The drawing under review shows one solid part. Ordinate dimensions are in mm from its lowest x, y, z. A direction names the side the tool comes from. Coordinates: 2 decimals unless noted, no trailing zeros. Order: outer loops, then holes, each group sorted by start corner. A loop starts at its lowest first (then second) coordinate and runs counter-clockwise, first axis right, second up. Notation, with made-up numbers: (31, -23.75) -> (60, -23.75) arc R8 cw to (60, -8.75) -> close; hole circle Ø11 at (16, 11). An arc over 180 degrees is marked (long way). Use a Markdown table: item, result. Add a question column.
Q1. Add section C-C (x = 24.5). State the section outline as (y, z) points.
Q2. Machinability: for the marked faces 1, 2, 3, 4 and 5, which of the approach directions +Z, -Z, +X, -X, +Y, -Y give a long, thin tool a straight path to every point of the face, cutting with its end or side? Answer none if there is none.
Q3. Add section B-B (y = 19). State the section outline as (x, z) points, then the cut area to 3 significant figures.
Q4. Add section A-A (z = 19). State the section outline as (x, y) points.
Q5. Wall thickness on probe 1 along X at (y, z) = (28.5, 8.5); probe 2 along X at (y, z) = (18.5, 32.5); probe 3 along Y at (x, z) = (53, 8.5): over which ranges is each line inside the solid? List them lowest first.
Q6. Insertion check: pin 1 (5.5 mm diameter, centred on x = 77, z = 25, fed in from -Y); pin 2 (5 mm diameter, centred on x = 9, y = 18.5, fed in from -Z); pin 3 (2 mm diameter, centred on x = 10, y = 26, fed in from +Z). Each pin has a flat end and moves straight along its axis. Give the tip position at first contact, or say it passes through.
Q7. Add section D-D (z = 9.5). State the section outline as (x, y) points, then the cut area to 3 significant figures.
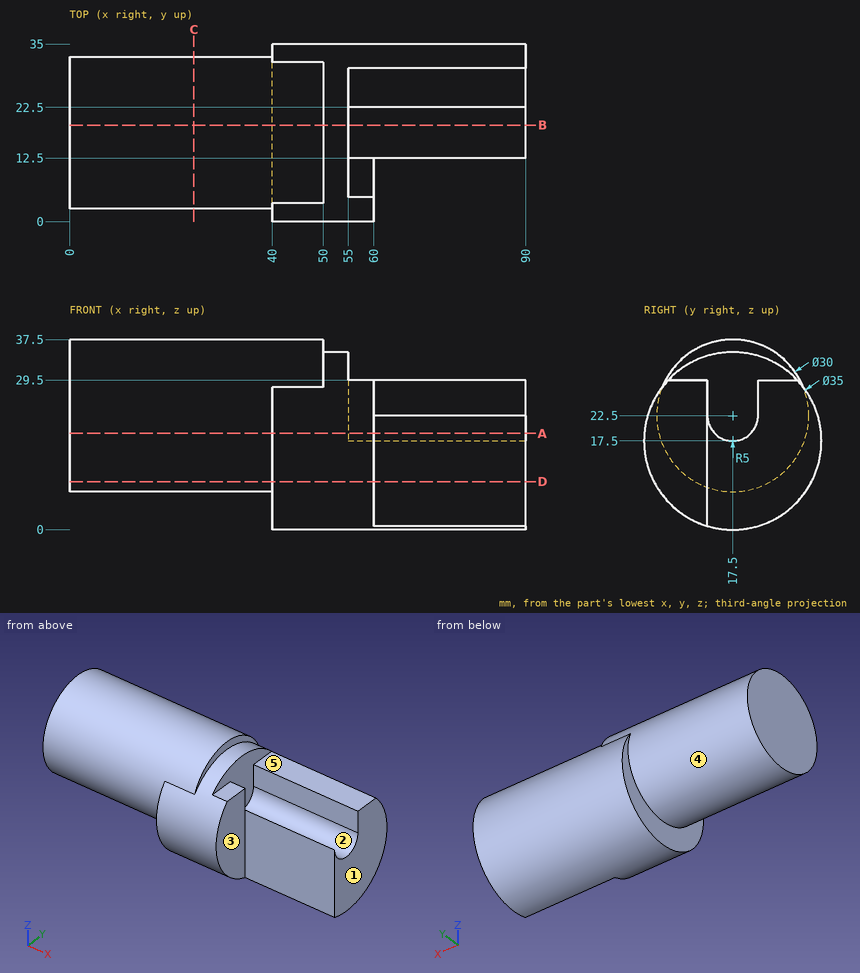
Established:
| question | item | result |
|---|---|---|
| 1 | outline | circle Ø30 at (17.5, 22.5) |
| 2 | face 1 | +Z, -Z, +X, +Y, -Y |
| 2 | face 2 | +Z, +X |
| 2 | face 3 | +Z, -Z, +X, -Y |
| 2 | face 4 | -X |
| 2 | face 5 | +Z, +X, +Y, -Y |
| 3 | outline | (0, 7.58) -> (40, 7.58) -> (40, 0.06) -> (90, 0.06) -> (90, 17.73) -> (55, 17.73) -> (55, 34.94) -> (50, 34.94) -> (50, 37.42) -> (0, 37.42) -> close |
| 3 | area | 2,360 mm^2 |
| 4 | outline | (0, 2.91) -> (40, 2.91) -> (40, 0.06) -> (60, 0.06) -> (60, 12.5) -> (90, 12.5) -> (90, 13.93) -> (55, 13.93) -> (55, 21.07) -> (90, 21.07) -> (90, 34.94) -> (40, 34.94) -> (40, 32.09) -> (0, 32.09) -> close |
| 5 | probe 1 | 40 to 90 |
| 5 | probe 2 | 0 to 55 |
| 5 | probe 3 | 2.49 to 32.51 |
| 6 | pin 1 | y = 12.5 |
| 6 | pin 2 | z = 7.5 |
| 6 | pin 3 | z = 35.49 |
| 7 | outline | (0, 10.02) -> (40, 10.02) -> (40, 1.94) -> (60, 1.94) -> (60, 12.5) -> (90, 12.5) -> (90, 33.06) -> (40, 33.06) -> (40, 24.98) -> (0, 24.98) -> close |
| 7 | area | 1,840 mm^2 |
